Geometry check sheet. Reference: the model listing, model coordinates, mm. A direction names the side the tool comes from. Round coordinates to 2 decimals unless told otherwise and drop trailing zeros. Order: outer loops, then holes, each group sorted by start corner. A loop starts at its lowest first (then second) coordinate and runs counter-clockwise, first axis right, second up.
(1) Set-up check for faces 1 (the face through (-1.38, 6.2, -25.04)), 2 (the face through (-11.34, -3.22, 92.84)), 3 (the face through (11.34, -3.22, 92.84)): record each of +Z, -Z, +X, -X, +Y, -Y from which the full face is reachable in a straight line by a thin tool's end or side.
(2) Cross-section at B-B on x = 21.5. Enter the section's corners in (y, z), and give its area (3 significant figures).
(3) Thickness scan on L1, parallel to X at y = 4.25, z = 206; L2, parallel to Z at x = 6, y = -11; L3, parallel to X at y = -6.25, z = 38.5. Record the ranges inside material, lowest first.
(4) Cross-section at D-D on z = -10.5. Enter the section's corners in (x, y).
(5) Cross-section at C-C on y = 8.75. Enter the section's corners in (x, z).
(6) Gauge pin test, flat ends, axial feed: P1, Ø10, axis at y = -6.5, z = 197.5, coming from the +X side; P2, Ø2, axis at x = -10, y = 9.5, coming from the -Z side; P3, Ø3, axis at x = 0.5, z = 72.5, coming from the -Y side. Record the tip position at first contact, or that the pin passes through.
from build123d import *

# Parameters (mm, degrees)
F0_W        = 50.8
F0_H        = 25.4
F1_DEPTH    = 12.7
F2_R        = 6.35
F3_DEPTH    = 50.8
F4_W        = 35.56
F4_H        = 12.7
F5_DEPTH    = 220.98
F6_SIZE2    = 12.69999
F6_SIZE     = 6.34999
F6_2_SIZE2  = 12.69999
F6_2_SIZE   = 6.34999
F7_T1_DEPTH = 317.8886374297
F7_T3_DEPTH = 317.8886374297
F7_T5_DEPTH = 317.8886374297
F7_T7_DEPTH = 317.8886374297
F8_SIZE2    = 7.62
F8_SIZE     = 7.62


# Not quite as in the source:
# - a fillet or chamfer that OpenCascade refuses, or shapes differently, is made with other operations: its cross-section is extruded or revolved along the edge and cut away or added
# - a fillet or chamfer is up to 0.001 mm smaller than in the source, because OpenCascade refuses the exact size


with BuildPart() as f1:
    # F0 (on Top) → F1 (new body)
    with BuildSketch(Plane.XY):
        Rectangle(F0_W, F0_H)
    extrude(amount=F1_DEPTH)

    # F2 (on face) → F3 (join)
    with BuildSketch(Plane(origin=(0, 0, 0), x_dir=(1, 0, 0), z_dir=(0, 0, -1))):
        Circle(F2_R)
    extrude(amount=F3_DEPTH)

    # F4 (on face) → F5 (join)
    with BuildSketch(Plane.XY.offset(12.7)):
        Rectangle(F4_W, F4_H)
    extrude(amount=F5_DEPTH)

    # F6 (size 6.35 and 12.7 in the source; OpenCascade refuses exactly that, so slightly less here)
    f6_edges = [f1.edges().sort_by_distance(p)[0] for p in [
        (17.78, -6.35, 123.19),
        (17.78, 6.35, 123.19),
    ]]
    f6_side = f1.faces().sort_by_distance((17.78, 0, 123.19))[0]
    chamfer(f6_edges, length=F6_SIZE, length2=F6_SIZE2, reference=f6_side)

    # F6#2 (size 6.35 and 12.7 in the source; OpenCascade refuses exactly that, so slightly less here)
    f6_2_edges = [f1.edges().sort_by_distance(p)[0] for p in [
        (-17.78, 6.35, 123.19),
        (-17.78, -6.35, 123.19),
    ]]
    f6_2_side = f1.faces().sort_by_distance((-17.78, 0, 123.19))[0]
    chamfer(f6_2_edges, length=F6_2_SIZE, length2=F6_2_SIZE2, reference=f6_2_side)

    # F7: chamfer of 7.62 x 58.42 on 4 edges, made by hand

    # F7_s2 → F7_t1 (cut)
    with BuildSketch(Plane(origin=(150.0381483816, -75.0190151206, 0), x_dir=(0, 0, 1), z_dir=(-0.8944273319, 0.4472133138, 0))):
        Polygon((175.26, 7.9514616635), (233.68, 0.3314616635), (233.68, 7.9514616635), align=None)
    extrude(amount=F7_T1_DEPTH, mode=Mode.SUBTRACT)

    # F7_s4 → F7_t3 (cut)
    with BuildSketch(Plane(origin=(150.0381483816, 75.0190151206, 0), x_dir=(0, 0, 1), z_dir=(-0.8944273319, -0.4472133138, 0))):
        Polygon((175.26, -7.9514616635), (233.68, -0.3314616635), (233.68, -7.9514616635), align=None)
    extrude(amount=F7_T3_DEPTH, mode=Mode.SUBTRACT)

    # F7_s6 → F7_t5 (cut)
    with BuildSketch(Plane(origin=(-150.0381483816, 75.0190151206, 0), x_dir=(0, 0, 1), z_dir=(0.8944273319, -0.4472133138, 0))):
        Polygon((175.26, 7.9514616635), (233.68, 0.3314616635), (233.68, 7.9514616635), align=None)
    extrude(amount=F7_T5_DEPTH, mode=Mode.SUBTRACT)

    # F7_s8 → F7_t7 (cut)
    with BuildSketch(Plane(origin=(-150.0381483816, -75.0190151206, 0), x_dir=(0, 0, 1), z_dir=(0.8944273319, 0.4472133138, 0))):
        Polygon((175.26, -7.9514616635), (233.68, -0.3314616635), (233.68, -7.9514616635), align=None)
    extrude(amount=F7_T7_DEPTH, mode=Mode.SUBTRACT)

    # F8
    f8_edges = [f1.edges().sort_by_distance(p)[0] for p in [
        (-25.4, -12.7, 6.35),
        (25.4, -12.7, 6.35),
        (25.4, 12.7, 6.35),
        (-25.4, 12.7, 6.35),
    ]]
    chamfer(f8_edges, length=F8_SIZE, length2=F8_SIZE2)


solid = f1.part
Found:
1. face 1: -Z
1. face 2: +Z, -X, -Y
1. face 3: +Z, +X, -Y
2. outline: (-8.98, 0) - (8.98, 0) - (8.98, 12.7) - (-8.98, 12.7) - close
2. area: 228 mm2
3. L1: x = -0.31 to 0.31
3. L2: z = 0 to 12.7
3. L3: x = -5.28 to 5.28
4. outline: circle Ø12.7 at (0, 0)
5. outline: (-21.73, 0) - (21.73, 0) - (21.73, 12.7) - (-21.73, 12.7) - close
6. P1: stops at x = 8.4
6. P2: stops at z = 0
6. P3: stops at y = -6.35
